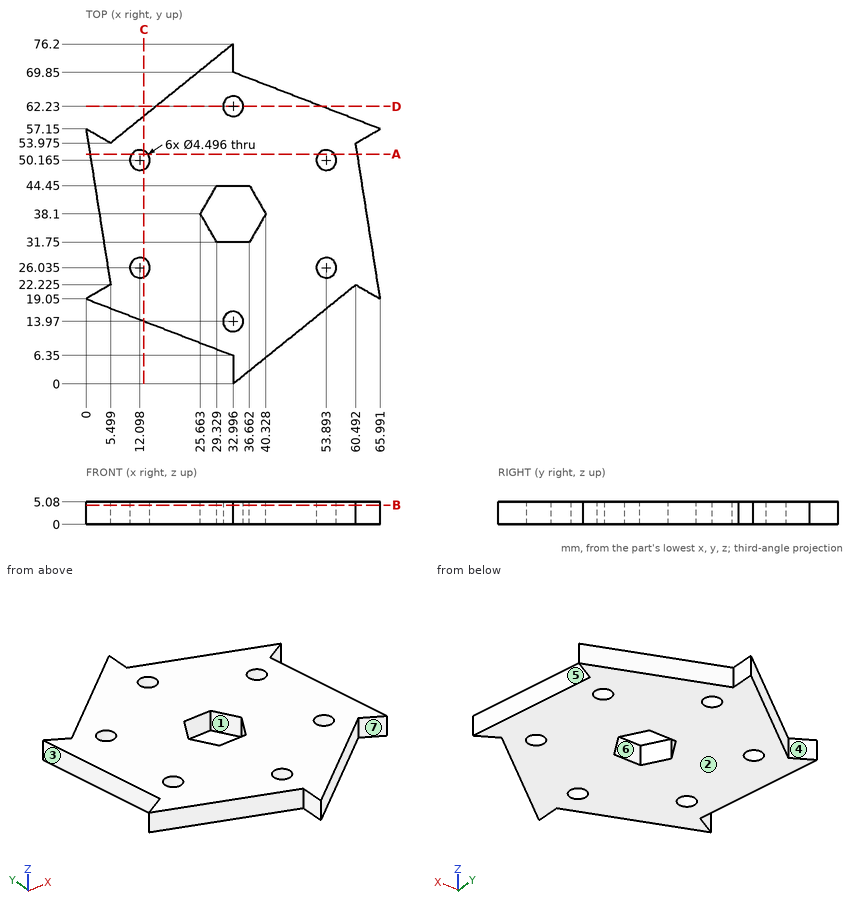
Study the drawing (mm; zero at the part's minimum x, y, z) and answer. A direction names the side the tool comes from. Give positions to 0.01 mm unless a question says otherwise; leave off trailing zeros. Loops run counter-clockwise (first coordinate to the right, second up) from the corner with the lowest first, then second, coordinate; pieces in that order, holes last. Notation, with made-up numbers: (23.5, 52.25) - (79.5, 52.25) arc R13 ccw to (79.5, 59.25) - close; hole circle Ø3 at (55, 38.25). An arc over 180 degrees is marked (long way). Use CSV: the item, a comma, the result in double quotes. Start each with the question number.
(1) Find section D-D, the plane y = 62.23. Determine the outline of the cut face in (x, z).
(2) Find section C-C, the plane x = 13. Determine the outline of the cut face in (y, z) (1 decimal).
(3) A tool of negligible diameter and unlimited length cuts with its end or side. For the marked faces 4, 5, 6 and 7, from which of +Z, -Z, +X, -X, +Y, -Y can it reach the whole face along a straight path? Write none if from no direction.
(4) Determine the mould class of the marked faces 1, 2 and 3 for opening direction X: released by +X, released by -X, zero draft, split by the parting line, or undercut.
(5) Each of these flat-tipped pins is pushed along its axis until it touches: pin 1 (3 mm diameter, centred on y = 40.5, z = 1.5, fed in from -X) (1 decimal); pin 2 (4 mm diameter, centred on x = 53.89, y = 26.04, fed in from -Z); pin 3 (2.5 mm diameter, centred on y = 3.5, z = 1.5, fed in from -X); pin 4 (2 mm diameter, centred on x = 18, z = 4.5, fed in from +Y). Where does it stop, or does it pass through?
(6) Find section B-B, the plane z = 4.3. Count the separate pieces of the cut face and the enclosed holes in it, plus the area to 3 significant figures.
(7) Find the intervals of material crossed by L1, parallel to X at y = 49, z = 4.8 (1 decimal); L2, parallel to Y at x = 36.5, z = 3.25; L3, parallel to X at y = 21, z = 2.35 (1 decimal), in increasing order.
(8) Find section A-A, the plane y = 51.5. Determine the outline of the cut face in (x, z) (1 decimal), plus the area to 3 significant figures.
Results found:
1,outline,"(15.71, 0) - (30.75, 0) - (30.75, 5.08) - (15.71, 5.08) - close; (35.24, 0) - (52.79, 0) - (52.79, 5.08) - (35.24, 5.08) - close"
2,outline,"(14, 0) - (24, 0) - (24, 5.1) - (14, 5.1) - close; (28.1, 0) - (48.1, 0) - (48.1, 5.1) - (28.1, 5.1) - close; (52.2, 0) - (60, 0) - (60, 5.1) - (52.2, 5.1) - close"
3,face 4,"+Z, -Z, +Y"
3,face 5,"+Z, -Z, +X"
3,face 6,"+Z, -Z"
3,face 7,"+Z, -Z, -Y"
4,face 1,"undercut"
4,face 2,"zero draft"
4,face 3,"released by -X"
5,pin 1,"x = 2.4"
5,pin 2,"through"
5,pin 3,"x = 33"
5,pin 4,"y = 64.89"
6,separate pieces,"1"
6,enclosed holes,"7"
6,area,"2,910 mm^2"
7,L1,"1.3 to 10.2, 14 to 52, 55.8 to 61.3"
7,L2,"2.83 to 31.75, 44.45 to 68.5"
7,L3,"3.4 to 59, 62.6 to 65.7"
8,outline,"(0.9, 0) - (10.3, 0) - (10.3, 5.1) - (0.9, 5.1) - close; (13.9, 0) - (52.1, 0) - (52.1, 5.1) - (13.9, 5.1) - close; (55.7, 0) - (60.9, 0) - (60.9, 5.1) - (55.7, 5.1) - close"
8,area,"268 mm^2"
